from build123d import *

# Parameters (mm, degrees)
STOCK_HORN_ATTACHMENT_START         = 15
STOCK_HORN_ATTACHMENT_PROFILE_R     = 11
STOCK_HORN_ATTACHMENT_DEPTH         = 3
FINGER_ARM_START                    = 15
FINGER_ARM_PROFILE_W                = 27
FINGER_ARM_PROFILE_H                = 10
FINGER_ARM_DEPTH                    = 3
DESCENDING_CONTACT_FINGER_PROFILE_W = 12
DESCENDING_CONTACT_FINGER_PROFILE_H = 3
DESCENDING_CONTACT_FINGER_DEPTH     = 18
HORN_CENTER_ACCESS_START            = -50
HORN_CENTER_ACCESS_PROFILE_R        = 3
HORN_CENTER_ACCESS_DEPTH            = 85.263683398
HORN_SCREWS_START                   = -50
HORN_SCREWS_PROFILE_R               = 1.1
HORN_SCREWS_DEPTH                   = 85.263683398
CONTACT_PAD_KEEPER_START            = -50
CONTACT_PAD_KEEPER_PROFILE_R        = 0.85
CONTACT_PAD_KEEPER_DEPTH            = 85.263683398


with BuildPart() as part:
    # Stock_horn_attachment_profile → Stock_horn_attachment (new body)
    with BuildSketch(Plane.XY.offset(STOCK_HORN_ATTACHMENT_START)):
        Circle(STOCK_HORN_ATTACHMENT_PROFILE_R)
    extrude(amount=STOCK_HORN_ATTACHMENT_DEPTH)

    # Finger_arm_profile → Finger_arm (add)
    with BuildSketch(Plane.XY.offset(FINGER_ARM_START)):
        with Locations((13.5, -2)):
            Rectangle(FINGER_ARM_PROFILE_W, FINGER_ARM_PROFILE_H)
    extrude(amount=FINGER_ARM_DEPTH)

    # Descending_contact_finger_profile → Descending_contact_finger (add)
    with BuildSketch(Plane.XY):
        with Locations((21, -5.5)):
            Rectangle(DESCENDING_CONTACT_FINGER_PROFILE_W, DESCENDING_CONTACT_FINGER_PROFILE_H)
    extrude(amount=DESCENDING_CONTACT_FINGER_DEPTH)

    # Horn_center_access_profile → Horn_center_access (cut, through all)
    with BuildSketch(Plane.XY.offset(HORN_CENTER_ACCESS_START)):
        Circle(HORN_CENTER_ACCESS_PROFILE_R)
    extrude(amount=HORN_CENTER_ACCESS_DEPTH, mode=Mode.SUBTRACT)

    # Horn_screws_profile → Horn_screws (cut, through all)
    with BuildSketch(Plane.XY.offset(HORN_SCREWS_START)):
        with Locations((0, -7)):
            Circle(HORN_SCREWS_PROFILE_R)
        with Locations((0, 7)):
            Circle(HORN_SCREWS_PROFILE_R)
        with Locations((-7, 0)):
            Circle(HORN_SCREWS_PROFILE_R)
        with Locations((7, 0)):
            Circle(HORN_SCREWS_PROFILE_R)
    extrude(amount=HORN_SCREWS_DEPTH, mode=Mode.SUBTRACT)

    # Contact_pad_keeper_profile → Contact_pad_keeper (cut, through all)
    with BuildSketch(Plane.XY.offset(CONTACT_PAD_KEEPER_START)):
        with Locations(Location((18, -5.5, 0), (0, 0, 180))):
            Circle(CONTACT_PAD_KEEPER_PROFILE_R)
        with Locations(Location((24, -5.5, 0), (0, 0, 180))):
            Circle(CONTACT_PAD_KEEPER_PROFILE_R)
    extrude(amount=CONTACT_PAD_KEEPER_DEPTH, mode=Mode.SUBTRACT)


solid = part.part
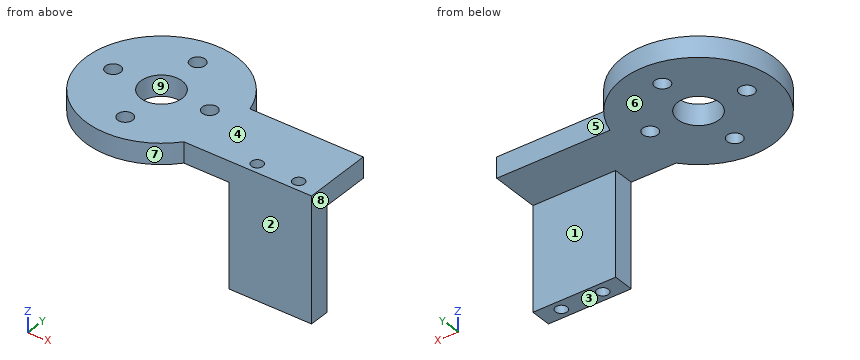
Read the model definition and answer for the solid it produces. Units are mm, in the model's axes. Face numbers are marked on the shaded views. A direction names the side the tool comes from. Round coordinates to 2 decimals unless told otherwise and drop trailing zeros. Write each loop counter-clockwise with the first axis right and the second up, starting at its lowest first coordinate (ties: lowest second). Pieces come first, ordered by that corner, then holes. Notation, with made-up numbers: M -27.5,-11 L -23.5,-11 A20 ccw -23.5,3 Z; hole C -29.75,-2.75 d2. An arc over 180 degrees is marked long. Use a Markdown table: item, result.
1) The part is cut by section C-C (x = 0). Write down the section's boundary in (y, z).
Answers follow:
| item | result |
|---|---|
| outline | M -11,15 L -8.1,15 L -8.1,18 L -11,18 Z; M -5.9,15 L -3,15 L -3,18 L -5.9,18 Z; M 3,15 L 5.9,15 L 5.9,18 L 3,18 Z; M 8.1,15 L 11,15 L 11,18 L 8.1,18 Z |
2) A tool of negligible diameter and unlimited length cuts with its end or side. For the marked faces 1, 2, 3, 4 and 5, from which of +Z, -Z, +X, -X, +Y, -Y can it reach the whole face along a straight path? Write none if from no direction.
Answers follow:
| item | result |
|---|---|
| face 1 | -Z, +X, -X, +Y |
| face 2 | +Z, -Z, +X, -Y |
| face 3 | -Z, +X, -X, +Y, -Y |
| face 4 | +Z, +X, -X, +Y, -Y |
| face 5 | +Z, -Z, +X, +Y |
3) The part is cut by section B-B (z = 6). Write down the section's boundary in (x, y).
Answers follow:
| item | result |
|---|---|
| outline | M 15,-7 L 27,-7 L 27,-4 L 15,-4 Z; hole C 18,-5.5 d1.7; hole C 24,-5.5 d1.7 |
4) For a pull along X with two mould halves and no side action, classify the marked faces 6, 7, 8 and 9 as pulls with the +X half, pulls with the -X half, needs draft (parallel to the pull), parting line crosses it, or undercut.
Answers follow:
| item | result |
|---|---|
| face 6 | needs draft |
| face 7 | parting line crosses it |
| face 8 | pulls with the +X half |
| face 9 | undercut |
5) Flat-ended cylindrical pins translate along their axes: pin 1 (8 mm diameter, centred on x = 0, y = 0, fed in from -Z); pin 2 (1.5 mm diameter, centred on y = -2, z = 6.5, fed in from -X); pin 3 (5.5 mm diameter, centred on x = 17, z = 9.5, fed in from -Y); pin 4 (6 mm diameter, centred on x = 18.5, z = 10.5, fed in from +Y). Find the tip coordinate at first contact, or state that the pin passes through.
Answers follow:
| item | result |
|---|---|
| pin 1 | stops at z = 15 |
| pin 2 | passes through |
| pin 3 | stops at y = -7 |
| pin 4 | stops at y = -4 |
6) The part is cut by section D-D (y = 7). Write down the section's boundary in (x, z), plus the area to 3 significant figures.
Answers follow:
| item | result |
|---|---|
| outline | M -8.49,15 L -1.1,15 L -1.1,18 L -8.49,18 Z; M 1.1,15 L 8.49,15 L 8.49,18 L 1.1,18 Z |
| area | 44.3 mm2 |
7) The part is cut by section A-A (x = 24). Write down the section's boundary in (y, z), plus the area to 3 significant figures.
Answers follow:
| item | result |
|---|---|
| outline | M -7,0 L -6.35,0 L -6.35,18 L -7,18 Z; M -4.65,0 L -4,0 L -4,15 L 3,15 L 3,18 L -4.65,18 Z |
| area | 44.4 mm2 |
8) Straight lines are drawn through the part: line 1 along X through (y, z) = (0, 16.75); line 2 along Y through (x, z) = (0, 16.5); line 3 along Y through (x, z) = (24, 11). For each, find the intervals that lie inside material, in ascending order. Write a range as [from, to].
Answers follow:
| item | result |
|---|---|
| line 1 | x = [-11, -8.1], [-5.9, -3], [3, 5.9], [8.1, 27] |
| line 2 | y = [-11, -8.1], [-5.9, -3], [3, 5.9], [8.1, 11] |
| line 3 | y = [-7, -6.35], [-4.65, -4] |
